Build history of the part. All positions in model axes, mm. A direction names the side the tool comes from. Give positions to 0.01 mm unless a question says otherwise; leave off trailing zeros. Order: outer loops, then holes, each group sorted by start corner. A loop starts at its lowest first (then second) coordinate and runs counter-clockwise, first axis right, second up. Notation, with made-up numbers: (-22.75, 0.25) - (-7.75, 0.25) arc R20 ccw to (-7.75, 20.25) - close; hole circle Ø7 at (59, 33.25). An arc over 180 degrees is marked (long way). One line per item, written item: value.
```python
from build123d import *

# Parameters (mm, degrees)
SKETCH1_W           = 10
SKETCH1_H           = 10
SKETCH1_W_2         = 8
SKETCH1_H_2         = 8
BOSS_EXTRUDE1_DEPTH = 200
FILLET2_R           = 1
SKETCH2_R           = 2.2
SKETCH2_R_2         = 2.25
CUT_EXTRUDE1_DEPTH  = 201.31225624


with BuildPart() as part:
    # Sketch1 → Boss-Extrude1 (new body)
    with BuildSketch(Plane(origin=(0, 0, 0), x_dir=(1, 0, 0), z_dir=(0, 1, 0))):
        Rectangle(SKETCH1_W, SKETCH1_H)
        Rectangle(SKETCH1_W_2, SKETCH1_H_2, mode=Mode.SUBTRACT)
    extrude(amount=BOSS_EXTRUDE1_DEPTH)

    # Fillet2
    fillet2_edges = [part.edges().sort_by_distance(p)[0] for p in [
        (4, 0, 0),
        (0, 0, -4),
        (-4, 0, 0),
        (0, 0, 4),
        (4, 200, 0),
        (0, 200, -4),
        (-4, 200, 0),
        (0, 200, 4),
    ]]
    fillet(fillet2_edges, radius=FILLET2_R - 0.0001)  # a hair under: the kernel refuses the full size

    # Sketch2 → Cut-Extrude1 (cut, through all)
    with BuildSketch(Plane.XY.offset(5)):
        with Locations((0, 5)):
            Circle(SKETCH2_R)
        with Locations((0, 195)):
            Circle(SKETCH2_R_2)
    extrude(amount=-CUT_EXTRUDE1_DEPTH, mode=Mode.SUBTRACT)


solid = part.part
```
(1) Pin check, flat tips, straight feed: P1, Ø5.5, axis at x = 0, y = 5, coming from the +Z side; P2, Ø3.5, axis at x = 0, y = 5, coming from the +Z side. Stop position of each tip, or through.
Completed:
P1: z = 5
P2: through
(2) Slice it at A-A, the plane x = 0. Count the separate pieces of the cut face and the enclosed holes in it, and give its area (3 significant figures).
Completed:
separate pieces: 6
enclosed holes: 0
area: 381 mm²
(3) Slice it at D-D, the plane y = 157.5. Give the cut face in (x, z).
Completed:
outline: (-5, -5) - (5, -5) - (5, 5) - (-5, 5) - close; hole (-4, -4) - (4, -4) - (4, 4) - (-4, 4) - close
(4) 3-axis set-ups, long thin cutter, end or side, ignore diameter. For faces 4 (the face through (0, 99, -4)), 5 (the face through (5, 99, 0)): which of +Z, -Z, +X, -X, +Y, -Y reach the whole face in a straight line?
Completed:
face 4: +Y, -Y
face 5: +Z, -Z, +X, +Y, -Y
(5) Slice it at C-C, the plane y = 5. Give the cut face in (x, z), and give its area (3 significant figures).
Completed:
outline: (-5, -5) - (-2.2, -5) - (-2.2, -4) - (-4, -4) - (-4, 4) - (-2.2, 4) - (-2.2, 5) - (-5, 5) - close; (2.2, -5) - (5, -5) - (5, 5) - (2.2, 5) - (2.2, 4) - (4, 4) - (4, -4) - (2.2, -4) - close
area: 27.2 mm²
(6) Drill centre lines: line 1 (Z direction, x = -2.5, y = 132); line 2 (Y direction, x = 0, z = 4.85). Where is each one in solid material? Low to high.
Completed:
line 1: -5 to -4, 4 to 5
line 2: 0.01 to 2.8, 7.2 to 192.75, 197.25 to 199.99
(7) Pull direction Z, two halves, no side cores. Call faces 1 (the face through (-5, 99, 0)), 2 (the face through (4, 99, 0)), 3 (the face through (0, 99, 5)): +Z half, -Z half, draft (parallel to the pull), parting line (faces both ways), or undercut.
Completed:
face 1: draft
face 2: undercut
face 3: +Z half
